Geometry: final body of the model. Coordinates: model frame, mm. Face numbers are marked on the shaded views. Give positions to 0.01 mm unless a question says otherwise; leave off trailing zeros. Write each loop counter-clockwise with the first axis right and the second up, starting at its lowest first coordinate (ties: lowest second). Pieces come first, ordered by that corner, then holes. Notation, with made-up numbers: (15, 78) -> (37, 78) arc R13 ccw to (37, 92) -> close; hole circle Ø2 at (-34, 45). An arc over 180 degrees is marked (long way). Answer as a JSON object with one key per item and string values.
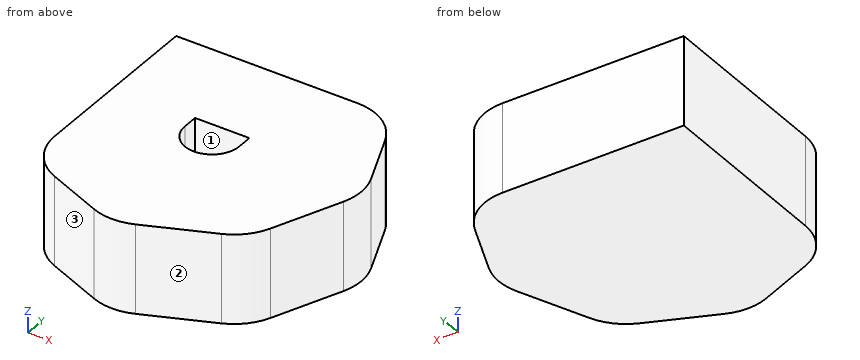
from build123d import *

# Parameters (mm, degrees)
F1_DEPTH = 10.414
F3_DEPTH = 1.27
F4_R     = 6.35
F6_ANGLE = 180


with BuildPart() as f1:
    # F0 (on Top) → F1 (new body)
    with BuildSketch(Plane.XY):
        Polygon((0, 17.960512), (-12.7, 12.7), (-12.7, -12.7), (12.7, -12.7), (17.960512, 0), (12.7, 12.7), align=None)
        with BuildLine():
            ThreePointArc((-3.175, 0), (0, 3.175), (3.175, 0))
            Line((3.175, 0), (3.175, -1.778))
            Line((3.175, -1.778), (-3.175, -1.778))
            Line((-3.175, -1.778), (-3.175, 0))
        make_face(mode=Mode.SUBTRACT)
    extrude(amount=F1_DEPTH)

    # F2 (on face) → F3 (join)
    with BuildSketch(Plane.XY.offset(10.414)):
        with BuildLine():
            ThreePointArc((3.175, 0), (0, 3.175), (-3.175, 0))
            Line((-3.175, 0), (-3.175, -1.778))
            Line((-3.175, -1.778), (3.175, -1.778))
            Line((3.175, -1.778), (3.175, 0))
        make_face()
    extrude(amount=-F3_DEPTH)

    # F4
    f4_edges = [f1.edges().sort_by_distance(p)[0] for p in [
        (12.7, -12.7, 5.207),
        (17.960512, 0, 5.207),
        (12.7, 12.7, 5.207),
        (0, 17.960512, 5.207),
        (-12.7, 12.7, 5.207),
    ]]
    fillet(f4_edges, radius=F4_R)


with BuildPart() as f1_1:
    # F6: moved
    add(f1.part.rotate(Axis((10.708487, 0, 0), (1, 0, 0)), F6_ANGLE))


solid = f1_1.part
Q1. Cut plane A-A (z = -5). Return the cut outline in (x, y) (3 decimals).
Values:
{"outline": "(-12.7, -8.457) arc R6.35 ccw to (-8.78, -14.324) -> (-2.43, -16.954) arc R6.35 ccw to (2.43, -16.954) -> (10.27, -13.707) arc R6.35 ccw to (13.707, -10.27) -> (16.954, -2.43) arc R6.35 ccw to (16.954, 2.43) -> (14.324, 8.78) arc R6.35 ccw to (8.457, 12.7) -> (-12.7, 12.7) -> close; hole (-3.175, 0) arc R3.175 ccw to (3.175, 0) -> (3.175, 1.778) -> (-3.175, 1.778) -> close"}
Q2. Material intervals for L1, parallel to X at y = 0.5, z = -6 (3 decimals); L2, parallel to Y at x = -2.5, z = -6; L3, parallel to Y at x = -10, z = -2.5, sorted ascending. Write a range as from..to.
Values:
{"L1": "-12.7..-3.175, 3.175..17.418", "L2": "-16.92..-1.96, 1.78..12.7", "L3": "-13.65..12.7"}
Q3. Cut plane B-B (x = 0). Return the cut outline in (y, z) (3 decimals).
Values:
{"outline": "(-17.437, -10.414) -> (12.7, -10.414) -> (12.7, 0) -> (1.778, 0) -> (1.778, -9.144) -> (-3.175, -9.144) -> (-3.175, 0) -> (-17.437, 0) -> close"}
Q4. First-contact query: P1, Ø5.5, axis at x = -0.5, y = 0.5, coming from the +Z side; P2, Ø1, axis at x = 1, z = -8.5, coming from the -Y side; P3, Ø1.5, axis at x = 12.5, z = -1.5, coming from the -Y side; P4, Ø4, axis at y = -9.5, z = -6, coming from the +X side. Flat tips, straight axial feed; report the tip coordinate or a pass-through.
Values:
{"P1": "z = 0", "P2": "y = -17.42", "P3": "y = -12.84", "P4": "x = 14.85"}
Q5. Cut plane D-D (x = 5.5). Return the cut outline in (y, z).
Values:
{"outline": "(-15.68, -10.41) -> (12.7, -10.41) -> (12.7, 0) -> (-15.68, 0) -> close"}
Q6. Mould query, pull axis X, two halves, no side actions, for the marked faces 1, 2 and 3. Classes: pulls with the +X half, pulls with the -X half, needs draft (parallel to the pull), parting line crosses it, or undercut.
Values:
{"face 1": "undercut", "face 2": "pulls with the +X half", "face 3": "pulls with the -X half"}
Q7. Cut plane C-C (y = -12.5). Return the cut outline in (x, z).
Values:
{"outline": "(-11.25, -10.41) -> (12.15, -10.41) -> (12.15, 0) -> (-11.25, 0) -> close"}
